For this review, take the finished solid that the model builds, in its own axes (mm). Face numbers are marked on the shaded views. A direction names the side the tool comes from. Round coordinates to 2 decimals unless told otherwise and drop trailing zeros. Order: outer loops, then holes, each group sorted by start corner. A loop starts at its lowest first (then second) coordinate and runs counter-clockwise, first axis right, second up. Notation, with made-up numbers: (73.25, -35.5) -> (131.25, -35.5) arc R25 cw to (131.25, -12.5) -> close; hole circle Ø5 at (86, 4.5). An arc over 180 degrees is marked (long way). Use a Markdown table: item, result. Add a question column.
1) Machinability: for the marked faces 1 and 2, which of the approach directions +Z, -Z, +X, -X, +Y, -Y give a long, thin tool a straight path to every point of the face, cutting with its end or side? Answer none if there is none.
2) Consider section C-C (x = -6). State the section outline as (y, z) points, plus the area to 3 significant figures.
3) Clearance check with flat-ended pins moving along their axes: P1, Ø2.5, axis at x = -7, y = 1.5, coming from the -Z side; P2, Ø3, axis at y = 3, z = 26.5, coming from the -X side. State where each tip first meets the part, or that it passes through.
4) Consider section A-A (y = 2.5). State the section outline as (x, z) points, plus the area to 3 significant figures.
5) Wall thickness on line 1 along Z through (x, y) = (-22.25, 2.6); line 2 along X through (y, z) = (0.3, -0.5); line 3 along Z through (x, y) = (-4.5, 1.3): over which ranges is each line inside the solid? List them lowest first. Write a range as [from, to].
6) Consider section B-B (z = -10). State the section outline as (x, y) points.
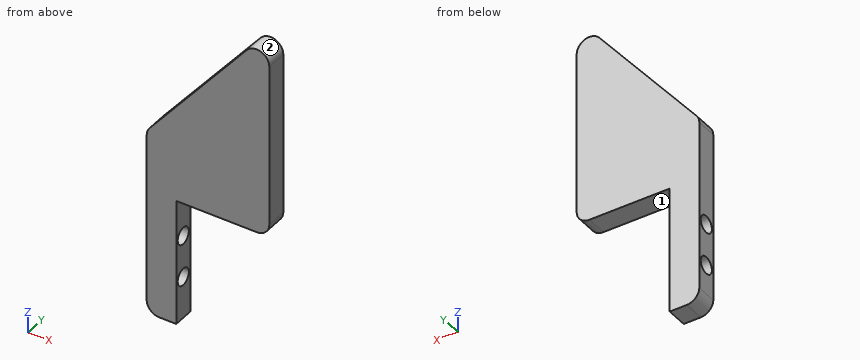
```python
from build123d import *

# Parameters (mm, degrees)
BOSS_EXTRUDE1_DEPTH = 5
SKETCH3_R           = 2
CUT_EXTRUDE2_DEPTH  = 20
FILLET2_R           = 3
FILLET3_R           = 3
FILLET4_R           = 3


with BuildPart() as part:
    # Sketch1 → Boss-Extrude1 (new body)
    with BuildSketch(Plane(origin=(0, 0, 0), x_dir=(1, 0, 0), z_dir=(0, 1, 0))):
        Polygon((2.364942178, -62.723244455), (-26.635057822, -27.094088406), (-26.635057822, 17.276755545), (-19.635057822, 17.276755545), (-19.635057822, -12.723244455), (2.364942178, -12.723244455), align=None)
    extrude(amount=BOSS_EXTRUDE1_DEPTH)

    # Sketch3 → Cut-Extrude2 (cut)
    with BuildSketch(Plane(origin=(-19.635057822, 0, 0), x_dir=(0, 0, -1), z_dir=(1, 0, 0))):
        with Locations((-2.723244455, 2.5)):
            Circle(SKETCH3_R)
        with Locations((7.276755545, 2.5)):
            Circle(SKETCH3_R)
    extrude(amount=-CUT_EXTRUDE2_DEPTH, mode=Mode.SUBTRACT)

    # Fillet2
    fillet2_edges = [part.edges().sort_by_distance(p)[0] for p in [
        (2.364942178, 2.5, 62.723244455),
    ]]
    fillet(fillet2_edges, radius=FILLET2_R)

    # Fillet3
    fillet3_edges = [part.edges().sort_by_distance(p)[0] for p in [
        (2.364942178, 2.5, 12.723244455),
        (-26.635057822, 2.5, -17.276755545),
    ]]
    fillet(fillet3_edges, radius=FILLET3_R)

    # Fillet4
    fillet4_edges = [part.edges().sort_by_distance(p)[0] for p in [
        (-26.635057822, 2.5, 27.094088406),
    ]]
    fillet(fillet4_edges, radius=FILLET4_R)


solid = part.part
```
Results list:
| question | item | result |
|---|---|---|
| 1 | face 1 | -Z, +X, +Y, -Y |
| 1 | face 2 | +Z, +Y, -Y |
| 2 | outline | (0, 12.72) -> (5, 12.72) -> (5, 52.45) -> (0, 52.45) -> close |
| 2 | area | 199 mm2 |
| 3 | P1 | z = 12.72 |
| 3 | P2 | x = -26.64 |
| 4 | outline | (-26.64, -14.28) arc R3 ccw to (-23.64, -17.28) -> (-19.64, -17.28) -> (-19.64, -9.28) -> (-26.64, -9.28) -> close; (-26.64, -5.28) -> (-19.64, -5.28) -> (-19.64, 0.72) -> (-26.64, 0.72) -> close; (-26.64, 4.72) -> (-19.64, 4.72) -> (-19.64, 12.72) -> (-0.64, 12.72) arc R3 ccw to (2.36, 15.72) -> (2.36, 54.29) arc R3 ccw to (-2.96, 56.18) -> (-25.96, 27.92) arc R3 ccw to (-26.64, 26.03) -> close |
| 4 | area | 1,070 mm2 |
| 5 | line 1 | [-17.28, -9.27], [-5.28, 0.73], [4.72, 32.48] |
| 5 | line 2 | [-26.64, -19.64] |
| 5 | line 3 | [12.72, 54.29] |
| 6 | outline | (-26.64, 0) -> (-19.64, 0) -> (-19.64, 5) -> (-26.64, 5) -> close |
